Work out the finished part from the listing and answer in its coordinate system (mm). A direction names the side the tool comes from. Coordinates: 2 decimals unless noted, no trailing zeros. Order: outer loops, then holes, each group sorted by start corner. A loop starts at its lowest first (then second) coordinate and runs counter-clockwise, first axis right, second up.
```python
from build123d import *

# Parameters (mm, degrees)
F0_W      = 38
F0_H      = 38
F0_W_2    = 34
F0_H_2    = 34
F0_W_3    = 30
F0_H_3    = 30
F1_DEPTH  = 5
F2_DEPTH  = 25
F4_DEPTH  = 25
F5_DEPTH  = 25
F6_R      = 2.5
F7_W      = 3
F7_H      = 25
F8_DEPTH  = 19
F9_DEPTH  = 19
F10_DEPTH = 6
F11_SIZE2 = 5.99999
F11_SIZE  = 2.99999
F12_SIZE2 = 2.99999
F12_SIZE  = 5.99999
F14_DEPTH = 3
F16_DEPTH = 3
F17_D     = 3
F18_DEPTH = 0.75
F19_DEPTH = 3
F20_DEPTH = 1.5
F21_W     = 2
F21_H     = 25
F22_DEPTH = 0.5


# Not quite as in the source:
# - a fillet or chamfer is up to 0.001 mm smaller than in the source, because OpenCascade refuses the exact size
# - a feature names something its author has since deleted; it is built from what else it names


with BuildPart() as f1:
    # F0 (on Top) → F1 (new body)
    with BuildSketch(Plane.XY):
        Rectangle(F0_W, F0_H)
        Rectangle(F0_W_2, F0_H_2, mode=Mode.SUBTRACT)
        Rectangle(F0_W_2, F0_H_2)
        Rectangle(F0_W_3, F0_H_3, mode=Mode.SUBTRACT)
        Rectangle(F0_W_3, F0_H_3)
    extrude(amount=F1_DEPTH)

    # F0 (on Top) → F2 (join)
    with BuildSketch(Plane.XY):
        Rectangle(F0_W_2, F0_H_2)
        Rectangle(F0_W_3, F0_H_3, mode=Mode.SUBTRACT)
    extrude(amount=-F2_DEPTH)

    # F3 (on face) → F4 (join)
    with BuildSketch(Plane.XY):
        Polygon((1.4142135624, 0), (0.7071067812, 0.7071067812), (0, 1.4142135624), (-13.5857864376, 15), (-15, 15), (-15, 13.5857864376), (-1.4142135624, 0), (-0.7071067812, -0.7071067812), (0, -1.4142135624), (13.5857864376, -15), (15, -15), (15, -13.5857864376), align=None)
        Polygon((0, 1.4142135624), (0.7071067812, 0.7071067812), (1.4142135624, 0), (15, 13.5857864376), (15, 15), (13.5857864376, 15), align=None)
    extrude(amount=-F4_DEPTH)

    # F3 (on face) → F5 (join)
    with BuildSketch(Plane.XY):
        Polygon((-0.7071067812, -0.7071067812), (-1.4142135624, 0), (-15, -13.5857864376), (-15, -15), (-13.5857864376, -15), (0, -1.4142135624), align=None)
    extrude(amount=-F5_DEPTH)

    # F6
    f6_edges = [f1.edges().sort_by_distance(p)[0] for p in [
        (0, 19, 5),
        (19, 0, 5),
        (-19, 0, 5),
        (0, -19, 5),
    ]]
    fillet(f6_edges, radius=F6_R)

    # F7 (on face) → F8 (join)
    with BuildSketch(Plane.XY.offset(5)):
        with Locations((-4.5, 0)):
            Rectangle(F7_W, F7_H)
    extrude(amount=F8_DEPTH)

    # F7 (on face) → F9 (join)
    with BuildSketch(Plane.XY.offset(5)):
        with Locations((4.5, 0)):
            Rectangle(F7_W, F7_H)
    extrude(amount=F9_DEPTH)

    # F7 (on face) → F10 (join)
    with BuildSketch(Plane.XY.offset(5)):
        with Locations((-7.5, 0)):
            Rectangle(F7_W, F7_H)
        with Locations((7.5, 0)):
            Rectangle(F7_W, F7_H)
    extrude(amount=F10_DEPTH)

    # F11 (size 3 and 6 in the source; OpenCascade refuses exactly that, so slightly less here)
    f11_edges = [f1.edges().sort_by_distance(p)[0] for p in [
        (-9, 0, 11),
    ]]
    f11_side = f1.faces().sort_by_distance((-7.5, 0, 11))[0]
    chamfer(f11_edges, length=F11_SIZE, length2=F11_SIZE2, reference=f11_side)

    # F12 (size 6 and 3 in the source; OpenCascade refuses exactly that, so slightly less here)
    f12_edges = [f1.edges().sort_by_distance(p)[0] for p in [
        (9, 0, 11),
    ]]
    f12_side = f1.faces().sort_by_distance((9, 0, 8))[0]
    chamfer(f12_edges, length=F12_SIZE, length2=F12_SIZE2, reference=f12_side)

    # F13 (on face) → F14 (join)
    with BuildSketch(Plane.YZ.offset(6)):
        with BuildLine():
            ThreePointArc((-12.5, 24), (0, 11.5), (12.5, 24))
            Line((12.5, 24), (5, 24))
            ThreePointArc((5, 24), (0, 19), (-5, 24))
            Line((-5, 24), (-12.5, 24))
        make_face()
        with BuildLine():
            Line((5, 24), (12.5, 24))
            ThreePointArc((12.5, 24), (0, 36.5), (-12.5, 24))
            Line((-12.5, 24), (-5, 24))
            ThreePointArc((-5, 24), (0, 29), (5, 24))
        make_face()
        with BuildLine():
            Line((1.5, 24), (5, 24))
            ThreePointArc((5, 24), (0, 29), (-5, 24))
            Line((-5, 24), (-1.5, 24))
            ThreePointArc((-1.5, 24), (0, 25.5), (1.5, 24))
        make_face()
        with BuildLine():
            Line((-1.5, 24), (1.5, 24))
            ThreePointArc((1.5, 24), (0, 25.5), (-1.5, 24))
        make_face()
    extrude(amount=-F14_DEPTH)

    # F15 (on face) → F16 (join)
    with BuildSketch(Plane(origin=(-6, 0, 0), x_dir=(0, -1, 0), z_dir=(-1, 0, 0))):
        with BuildLine():
            Line((-1.5, 24), (1.5, 24))
            ThreePointArc((1.5, 24), (0, 25.5), (-1.5, 24))
        make_face()
    extrude(amount=-F16_DEPTH)

    # F17 (through all)
    with Locations(Plane.YZ.offset(6)):
        with Locations((0, 24)):
            Hole(F17_D / 2)

    # F13 (on face) → F18 (cut, symmetric)
    with BuildSketch(Plane.YZ.offset(6)):
        with BuildLine():
            ThreePointArc((-5, 24), (0, 19), (5, 24))
            Line((5, 24), (1.5, 24))
            ThreePointArc((1.5, 24), (0, 22.5), (-1.5, 24))
            Line((-1.5, 24), (-5, 24))
        make_face()
        with BuildLine():
            Line((1.5, 24), (5, 24))
            ThreePointArc((5, 24), (0, 29), (-5, 24))
            Line((-5, 24), (-1.5, 24))
            ThreePointArc((-1.5, 24), (0, 25.5), (1.5, 24))
        make_face()
    extrude(amount=F18_DEPTH, both=True, mode=Mode.SUBTRACT)

    # F15 (on face) → F19 (join)
    with BuildSketch(Plane(origin=(-6, 0, 0), x_dir=(0, -1, 0), z_dir=(-1, 0, 0))):
        with BuildLine():
            Line((3.5, 24), (12.5, 24))
            ThreePointArc((12.5, 24), (0, 36.5), (-12.5, 24))
            Line((-12.5, 24), (-3.5, 24))
            Line((-3.5, 24), (-3.5, 26.0207259422))
            Line((-3.5, 26.0207259422), (0, 28.0414518843))
            Line((0, 28.0414518843), (3.5, 26.0207259422))
            Line((3.5, 26.0207259422), (3.5, 24))
        make_face()
        with BuildLine():
            Line((1.5, 24), (3.5, 24))
            Line((3.5, 24), (3.5, 26.0207259422))
            Line((3.5, 26.0207259422), (0, 28.0414518843))
            Line((0, 28.0414518843), (-3.5, 26.0207259422))
            Line((-3.5, 26.0207259422), (-3.5, 24))
            Line((-3.5, 24), (-1.5, 24))
            ThreePointArc((-1.5, 24), (0, 25.5), (1.5, 24))
        make_face()
    extrude(amount=-F19_DEPTH)

    # F15 (on face) → F20 (cut)
    with BuildSketch(Plane(origin=(-6, 0, 0), x_dir=(0, -1, 0), z_dir=(-1, 0, 0))):
        with BuildLine():
            Line((1.5, 24), (3.5, 24))
            Line((3.5, 24), (3.5, 26.0207259422))
            Line((3.5, 26.0207259422), (0, 28.0414518843))
            Line((0, 28.0414518843), (-3.5, 26.0207259422))
            Line((-3.5, 26.0207259422), (-3.5, 24))
            Line((-3.5, 24), (-1.5, 24))
            ThreePointArc((-1.5, 24), (0, 25.5), (1.5, 24))
        make_face()
        with BuildLine():
            Line((3.5, 21.9792740578), (3.5, 24))
            Line((3.5, 24), (1.5, 24))
            ThreePointArc((1.5, 24), (0, 22.5), (-1.5, 24))
            Line((-1.5, 24), (-3.5, 24))
            Line((-3.5, 24), (-3.5, 21.9792740578))
            Line((-3.5, 21.9792740578), (0, 19.9585481157))
            Line((0, 19.9585481157), (3.5, 21.9792740578))
        make_face()
    extrude(amount=-F20_DEPTH, mode=Mode.SUBTRACT)

    # F21 (on face) → F22 (cut, symmetric)
    with BuildSketch(Plane.XZ.offset(17)):
        with Locations((-2, -12.5)):
            Rectangle(F21_W, F21_H)
    extrude(amount=F22_DEPTH, both=True, mode=Mode.SUBTRACT)


solid = f1.part
```
1. The mould has two halves that part along X. Classify faces 1 (the flat face through (15, 0, -12)), 2 (the flat face through (0, 19, 1)), 3 (the flat face through (-17, 0, -12)): released by +X, released by -X, zero draft, split by the parting line, or undercut.
2. The part is cut by section B-B (z = -5). Determine the outline of the cut face in (x, y).
3. Consider probe 1 along Y at (x, z) = (-3.5, 24); probe 2 along Y at (x, z) = (-2, -3.5); probe 3 along X at (y, z) = (12, -3.5). Determine where each line is inside the solid, lowest interval first.
4. For faces 4 (the flat face through (8.302, -6.888, -12.325)), 5 (the cylindrical face through (5.63, -1.08, 19.12)), 6 (the flat face through (3, 0, 21)), determine the directions among +Z, -Z, +X, -X, +Y, -Y from which every point of the face is accessible in a straight line to the end or side of a thin tool.
5. The part is cut by section A-A (z = 8). Determine the outline of the cut face in (x, y), plus the area to 3 significant figures.
6. The part is cut by section C-C (x = 12). Determine the outline of the cut face in (y, z).
7. Flat-ended cylindrical pins translate along their axes: pin 1 (6 mm diameter, centred on y = -1, z = -4, fed in from -X); pin 2 (12.5 mm diameter, centred on y = -3.5, z = 26.5, fed in from +X); pin 3 (5 mm diameter, centred on x = -12, y = 5.5, fed in from -Z); pin 4 (2.5 mm diameter, centred on y = 0, z = 24, fed in from +X). Find the tip coordinate at first contact, or state that the pin passes through.
Worked out:
1. face 1: undercut
1. face 2: zero draft
1. face 3: released by -X
2. outline: (-17, -17) - (-3, -17) - (-3, -16.5) - (-1, -16.5) - (-1, -17) - (17, -17) - (17, 17) - (-17, 17) - close; hole (-15, -13.59) - (-1.41, 0) - (-15, 13.59) - close; hole (-13.59, -15) - (13.59, -15) - (0, -1.41) - close; hole (-13.59, 15) - (0, 1.41) - (13.59, 15) - close; hole (1.41, 0) - (15, -13.59) - (15, 13.59) - close
3. probe 1: y = -12.5 to -1.5, 1.5 to 12.5
3. probe 2: y = -16.5 to -15, -3.41 to -0.59, 0.59 to 3.41, 15 to 17
3. probe 3: x = -17 to -15, -13.41 to -10.59, 10.59 to 13.41, 15 to 17
4. face 4: -Z
4. face 5: +X
4. face 6: +Z, +Y, -Y
5. outline: (-7.5, -12.5) - (-3, -12.5) - (-3, 12.5) - (-7.5, 12.5) - close; (3, -12.5) - (7.5, -12.5) - (7.5, 12.5) - (3, 12.5) - close
5. area: 225 mm2
6. outline: (-19, 0) - (-17, 0) - (-17, -25) - (-15, -25) - (-15, 0) - (-13.41, 0) - (-13.41, -25) - (-10.59, -25) - (-10.59, 0) - (10.59, 0) - (10.59, -25) - (13.41, -25) - (13.41, 0) - (15, 0) - (15, -25) - (17, -25) - (17, 0) - (19, 0) - (19, 2.5) arc R2.5 ccw to (16.5, 5) - (-16.5, 5) arc R2.5 ccw to (-19, 2.5) - close
7. pin 1: stops at x = -17
7. pin 2: stops at x = 6
7. pin 3: stops at z = 0
7. pin 4: passes through
